from build123d import *

# Parameters (mm, degrees)
SKETCH1_W           = 6.35
SKETCH1_H           = 101.6
BOSS_EXTRUDE1_DEPTH = 457.2
SKETCH2_R           = 12.7
CUT_EXTRUDE1_DEPTH  = 467.602190566
CUT_EXTRUDE2_DEPTH  = 467.602190566


with BuildPart() as part:
    # Sketch1 → Boss-Extrude1 (new body)
    with BuildSketch(Plane(origin=(0, 0, 0), x_dir=(0, 0, -1), z_dir=(1, 0, 0))):
        with Locations((1.913371748, -42.180867605)):
            Rectangle(SKETCH1_W, SKETCH1_H)
    extrude(amount=BOSS_EXTRUDE1_DEPTH)

    # Sketch2 → Cut-Extrude1 (cut, through all)
    with BuildSketch(Plane(origin=(0, 0, -5.088371748), x_dir=(-1, 0, 0), z_dir=(0, 0, -1))):
        with Locations(Location((-355.6, -42.180867605, 0), (0, 0, 90))):
            Circle(SKETCH2_R)
        with Locations(Location((-101.6, -42.180867605, 0), (0, 0, 90))):
            Circle(SKETCH2_R)
    extrude(amount=-CUT_EXTRUDE1_DEPTH, mode=Mode.SUBTRACT)

    # Sketch3 → Cut-Extrude2 (cut, through all)
    with BuildSketch(Plane(origin=(0, 0, -5.088371748), x_dir=(-1, 0, 0), z_dir=(0, 0, -1))):
        with BuildLine():
            Line((-438.15, -4.080867605), (-402.680256121, -4.080867605))
            ThreePointArc((-402.680256121, -4.080867605), (-396.81362109, -8.000827809), (-398.190128061, -14.920995665))
            Line((-398.190128061, -14.920995665), (-433.659871939, -50.390739544))
            ThreePointArc((-433.659871939, -50.390739544), (-440.580039796, -51.767246515), (-444.5, -45.900611484))
            Line((-444.5, -45.900611484), (-444.5, -10.430867605))
            ThreePointArc((-444.5, -10.430867605), (-442.640128061, -5.940739544), (-438.15, -4.080867605))
        make_face()
        with BuildLine():
            Line((-398.190128061, -33.970995665), (-433.659871939, -69.440739544))
            ThreePointArc((-433.659871939, -69.440739544), (-435.03637891, -76.3609074), (-429.169743879, -80.280867605))
            Line((-429.169743879, -80.280867605), (-393.7, -80.280867605))
            ThreePointArc((-393.7, -80.280867605), (-389.209871939, -78.420995665), (-387.35, -73.930867605))
            Line((-387.35, -73.930867605), (-387.35, -38.461123726))
            ThreePointArc((-387.35, -38.461123726), (-391.269960204, -32.594488694), (-398.190128061, -33.970995665))
        make_face()
        with BuildLine():
            Line((-69.85, -73.930867605), (-69.85, -38.461123726))
            ThreePointArc((-69.85, -38.461123726), (-65.930039796, -32.594488694), (-59.009871939, -33.970995665))
            Line((-59.009871939, -33.970995665), (-23.540128061, -69.440739544))
            ThreePointArc((-23.540128061, -69.440739544), (-22.16362109, -76.3609074), (-28.030256121, -80.280867605))
            Line((-28.030256121, -80.280867605), (-63.5, -80.280867605))
            ThreePointArc((-63.5, -80.280867605), (-67.990128061, -78.420995665), (-69.85, -73.930867605))
        make_face()
        with BuildLine():
            Line((-23.540128061, -50.390739544), (-59.009871939, -14.920995665))
            ThreePointArc((-59.009871939, -14.920995665), (-60.38637891, -8.000827809), (-54.519743879, -4.080867605))
            Line((-54.519743879, -4.080867605), (-19.05, -4.080867605))
            ThreePointArc((-19.05, -4.080867605), (-14.559871939, -5.940739544), (-12.7, -10.430867605))
            Line((-12.7, -10.430867605), (-12.7, -45.900611484))
            ThreePointArc((-12.7, -45.900611484), (-16.619960204, -51.767246515), (-23.540128061, -50.390739544))
        make_face()
    extrude(amount=-CUT_EXTRUDE2_DEPTH, mode=Mode.SUBTRACT)


solid = part.part
Source: CAD feature listing. Evaluate the final solid. Frame: model axes, mm. A direction names the side the tool comes from. Coordinates: 2 decimals unless noted, no trailing zeros. Loops run counter-clockwise (first coordinate to the right, second up) from the corner with the lowest first, then second, coordinate; pieces in that order, holes last. Notation, with made-up numbers: (-32.5, 4) - (-28.5, 4) arc R13 cw to (-28.5, 22) - close; hole circle Ø4 at (17.5, 15). An arc over 180 degrees is marked (long way). One line per question, with ' | ' between items.
1) Section D-D, the plane x = 355.6. Return loops of the section in (y, z), then the cut area to 3 significant figures.
Report:
outline: (-92.98, -5.09) - (-54.88, -5.09) - (-54.88, 1.26) - (-92.98, 1.26) - close; (-29.48, -5.09) - (8.62, -5.09) - (8.62, 1.26) - (-29.48, 1.26) - close | area: 484 mm²
2) Section B-B, the plane y = -23.5. Return loops of the section in (x, z).
Report:
outline: (0, -5.09) - (12.7, -5.09) - (12.7, 1.26) - (0, 1.26) - close; (50.43, -5.09) - (406.77, -5.09) - (406.77, 1.26) - (50.43, 1.26) - close; (444.5, -5.09) - (457.2, -5.09) - (457.2, 1.26) - (444.5, 1.26) - close
3) Pull-direction query (Y, two-part tool) for faces 3 (the face through (225, -43, -5.088)), 4 (the face through (41.52, -51.46, -1.96)); classes: released by +Y, released by -Y, zero draft, split by the parting line, or undercut.
Report:
face 3: zero draft | face 4: undercut
4) Section A-A, the plane x = 423. Return loops of the section in (y, z), then the cut area to 3 significant figures.
Report:
outline: (-92.98, -5.09) - (-80.28, -5.09) - (-80.28, 1.26) - (-92.98, 1.26) - close; (-58.78, -5.09) - (-39.73, -5.09) - (-39.73, 1.26) - (-58.78, 1.26) - close; (-4.08, -5.09) - (8.62, -5.09) - (8.62, 1.26) - (-4.08, 1.26) - close | area: 282 mm²
5) Line query: line 1 along X through (y, z) = (-69.5, 1); line 2 along X through (y, z) = (-26.5, -1.5); line 3 along Y through (x, z) = (426.5, -1). Output: solid intervals per line, ascending.
Report:
line 1: x = 0 to 23.48, 69.85 to 387.35, 433.72 to 457.2 | line 2: x = 0 to 12.7, 47.43 to 409.77, 444.5 to 457.2 | line 3: y = -92.98 to -80.28, -62.28 to -43.23, -4.08 to 8.62
6) Set-up query: faces 1 (the face through (41.03, -32.9, -1.96)), 2 (the face through (225, -43, 1.262)). Return all of +Z, -Z, +X, -X, +Y, -Y with unobstructed straight access to the full face (end or side cutting, diameter ignored); none if empty.
Report:
face 1: +Z, -Z | face 2: +Z, +X, -X, +Y, -Y
7) Section C-C, the plane z = -3.25. Give the number of separate pieces and of enclosed holes in the cut face, then the cut area to 3 significant figures.
Report:
separate pieces: 1 | enclosed holes: 6 | area: 39,300 mm²
